from build123d import *

# Parameters (mm, degrees)
RESSALTO_EXTRUS_O1_DEPTH = 5
CORTE_EXTRUS_O1_DEPTH    = 6
ESBO_O3_R                = 2.262708027
ESBO_O3_R_2              = 2.332727501
ESBO_O3_W                = 27
ESBO_O3_H                = 18.8
CORTE_EXTRUS_O2_DEPTH    = 6


with BuildPart() as part:
    # Esboço1 → Ressalto-extrusão1 (new body)
    with BuildSketch(Plane.XY):
        Polygon((-26.727783806, -21.587024793), (-26.727783806, -1.587024793), (-31.727783806, -1.587024793), (-31.727783806, 8.412975207), (58.342216194, 8.412975207), (58.342216194, -1.587024793), (53.342216194, -1.587024793), (53.342216194, -21.587024793), align=None)
    extrude(amount=RESSALTO_EXTRUS_O1_DEPTH)

    # Esboço2 → Corte-extrusão1 (cut, through all)
    with BuildSketch(Plane.XY.offset(5)):
        Polygon((-31.727783806, 2.412975207), (-27.177783806, 2.412975207), (-27.177783806, 0.642975207), (-24.727783806, 0.642975207), (-24.727783806, 2.412975207), (-21.727783806, 2.412975207), (-21.727783806, 4.412975207), (-24.727783806, 4.412975207), (-24.727783806, 6.182975207), (-27.177783806, 6.182975207), (-27.177783806, 4.412975207), (-31.727783806, 4.412975207), align=None)
        Polygon((51.342216194, 4.412975207), (48.342216194, 4.412975207), (48.342216194, 2.412975207), (51.342216194, 2.412975207), (51.342216194, 0.642975207), (53.792216194, 0.642975207), (53.792216194, 2.412975207), (58.342216194, 2.412975207), (58.342216194, 4.412975207), (53.792216194, 4.412975207), (53.792216194, 6.182975207), (51.342216194, 6.182975207), align=None)
        Polygon((-26.727783806, -17.587024793), (-22.177783806, -17.587024793), (-22.177783806, -19.357024793), (-19.727783806, -19.357024793), (-19.727783806, -17.587024793), (-16.727783806, -17.587024793), (-16.727783806, -15.587024793), (-19.727783806, -15.587024793), (-19.727783806, -13.817024793), (-22.177783806, -13.817024793), (-22.177783806, -15.587024793), (-26.727783806, -15.587024793), align=None)
        Polygon((46.342216194, -15.587024793), (43.342216194, -15.587024793), (43.342216194, -17.587024793), (46.342216194, -17.587024793), (46.342216194, -19.357024793), (48.792216194, -19.357024793), (48.792216194, -17.587024793), (53.342216194, -17.587024793), (53.342216194, -15.587024793), (48.792216194, -15.587024793), (48.792216194, -13.817024793), (46.342216194, -13.817024793), align=None)
    extrude(amount=-CORTE_EXTRUS_O1_DEPTH, mode=Mode.SUBTRACT)

    # Esboço3 → Corte-extrusão2 (cut, through all)
    with BuildSketch(Plane.XY.offset(5)):
        with Locations((-19.474846983, -6.010345645)):
            Circle(ESBO_O3_R)
        with Locations((20.525153017, -6.010345645)):
            Circle(ESBO_O3_R_2)
        with Locations((0.525153017, -6.010345645)):
            Rectangle(ESBO_O3_W, ESBO_O3_H)
        with BuildLine():
            Line((34.525153017, 3.412975207), (39.342216194, 3.412975207))
            ThreePointArc((39.342216194, 3.412975207), (42.8777501, 1.948509113), (44.342216194, -1.587024793))
            Line((44.342216194, -1.587024793), (44.342216194, -11.587024793))
            ThreePointArc((44.342216194, -11.587024793), (42.8777501, -15.122558699), (39.342216194, -16.587024793))
            Line((39.342216194, -16.587024793), (34.525153017, -16.587024793))
            ThreePointArc((34.525153017, -16.587024793), (30.989619111, -15.122558699), (29.525153017, -11.587024793))
            Line((29.525153017, -11.587024793), (29.525153017, -1.587024793))
            ThreePointArc((29.525153017, -1.587024793), (30.989619111, 1.948509113), (34.525153017, 3.412975207))
        make_face()
    extrude(amount=-CORTE_EXTRUS_O2_DEPTH, mode=Mode.SUBTRACT)


solid = part.part
CAD build for the part. Positions are in the model's coordinates, mm. A direction names the side the tool comes from. Round coordinates to 2 decimals unless told otherwise and drop trailing zeros. Write each loop counter-clockwise with the first axis right and the second up, starting at its lowest first coordinate (ties: lowest second). Pieces come first, ordered by that corner, then holes. Notation, with made-up numbers: (-6, 39.5) -> (37, 39.5) arc R21 ccw to (37, 74.5) -> close; hole circle Ø2 at (71, -7.75). An arc over 180 degrees is marked (long way). Answer as a JSON object with one key per item and string values.
(1) Band-saw the part on D-D, the plane z = 1.3. Count the separate pieces of the cut face and the enclosed holes in it, then the cut area to 3 significant figures.
Reported:
{"separate pieces": "1", "enclosed holes": "4", "area": "1,570 mm^2"}
(2) Pin check, flat tips, straight feed: P1, Ø2, axis at y = -9.5, z = 2.5, coming from the -X side; P2, Ø0.6, axis at y = 3.5, z = 2.5, coming from the -X side; P3, Ø0.9, axis at y = -18.5, z = 1.5, coming from the +X side; P4, Ø1, axis at x = 44.5, y = -10.5, coming from the -Z side. Stop position of each tip, or through.
Reported:
{"P1": "stops at x = -26.73", "P2": "stops at x = -21.73", "P3": "stops at x = 53.34", "P4": "stops at z = 0"}
(3) Which spindle directions (+Z, -Z, +X, -X, +Y, -Y) get a long thin tool onto all of the face, cutting with end or side? Do faces 5 (the face through (4, 4, 0)), 6 (the face through (50, 2.413, 3)), 7 (the face through (48.792, -15, 3)), 8 (the face through (-29, 4.413, 3)). Say none if no direction does.
Reported:
{"face 5": "-Z, +X, -X, +Y, -Y", "face 6": "+Z, -Z, +X", "face 7": "+Z, -Z", "face 8": "+Z, -Z, -X"}
(4) Probe probe 1 along X at (y, z) = (-10.5, 3.7); probe 2 along Y at (x, z) = (51, 3.95); probe 3 along X at (y, z) = (5, 0.55). List the from-to ranges inside material, lowest first. Write a range as [from, to].
Reported:
{"probe 1": "x = [-26.73, -12.97], [14.03, 29.53], [44.34, 53.34]", "probe 2": "y = [-21.59, -17.59], [-15.59, 2.41], [4.41, 8.41]", "probe 3": "x = [-31.73, -27.18], [-24.73, 51.34], [53.79, 58.34]"}
(5) Two-plate mould, pull along Y, no slides. Class faces 1 (the face through (37, 3.413, 3)), 2 (the face through (13, 8.413, 2)), 3 (the face through (58.342, 0, 2)), 4 (the face through (14, -21.587, 2)): +Y half, -Y half, draft (parallel to the pull), parting line (faces both ways), or undercut.
Reported:
{"face 1": "undercut", "face 2": "+Y half", "face 3": "draft", "face 4": "-Y half"}
(6) Band-saw the part on C-C, the plane x = 42. List the corners of the cut face in (y, z).
Reported:
{"outline": "(-21.59, 0) -> (-15.82, 0) -> (-15.82, 5) -> (-21.59, 5) -> close; (2.65, 0) -> (8.41, 0) -> (8.41, 5) -> (2.65, 5) -> close"}
(7) Band-saw the part on B-B, the plane x = 10. List the corners of the cut face in (y, z).
Reported:
{"outline": "(-21.59, 0) -> (-15.41, 0) -> (-15.41, 5) -> (-21.59, 5) -> close; (3.39, 0) -> (8.41, 0) -> (8.41, 5) -> (3.39, 5) -> close"}
(8) Band-saw the part on A-A, the plane x = -23. List the corners of the cut face in (y, z).
Reported:
{"outline": "(-21.59, 0) -> (-17.59, 0) -> (-17.59, 5) -> (-21.59, 5) -> close; (-15.59, 0) -> (2.41, 0) -> (2.41, 5) -> (-15.59, 5) -> close; (4.41, 0) -> (8.41, 0) -> (8.41, 5) -> (4.41, 5) -> close"}
